Autodesk Inventor part; units mm, degrees
ref_plane "YZ Plane" through (0, 0, 0) normal (1, 0, 0) x (0, 1, 0)
ref_plane "XZ Plane" through (0, 0, 0) normal (0, 1, 0) x (-1, 0, 0)
ref_plane "XY Plane" through (0, 0, 0) normal (0, 0, 1) x (1, 0, 0)
sketch "Sketch1" plane through (0, 0, 0) normal (0, 0, 1) x (1, 0, 0)
  arc A0 (-6.0005, 54.2016) -> (-16.0004, 64.2461) centre (-16.0004, 54.2461) ccw construction
  line L0 (-16.0004, 64.2461) -> (-44.425, 64.2461) construction
  line L1 (-44.425, 64.2461) -> (-109.442, 0.9553) construction
  line L2 (-109.442, 0.9553) -> (-102.1149, -16.5964) construction
  arc A1 (-102.1149, -16.5964) -> (-98.2137, -18.2187) centre (-99.3465, -15.4407) ccw construction
  arc A2 (-98.2137, -18.2187) -> (-94.934, -16.1156) centre (-102.2552, -8.3072) ccw construction
  arc A3 (-90.1342, -27.6135) -> (-94.934, -16.1156) centre (-85.3155, -18.8511) ccw construction
  arc A4 (-90.1342, -27.6135) -> (-93.9357, -28.4666) centre (-89.7305, -38.3096) ccw construction
  arc A5 (-93.9357, -28.4666) -> (-95.5255, -32.381) centre (-92.7571, -31.2253) ccw construction
  line L3 (-95.5255, -32.381) -> (-88, -50.4082) construction
  line L4 (-88, -50.4082) -> (88, -50.4082) construction
  line L5 (88, -50.4082) -> (95.5255, -32.381) construction
  arc A6 (95.5255, -32.381) -> (93.9357, -28.4666) centre (92.7571, -31.2253) ccw construction
  arc A7 (93.9357, -28.4666) -> (90.1342, -27.6135) centre (89.7305, -38.3096) ccw construction
  arc A8 (94.934, -16.1156) -> (90.1342, -27.6135) centre (85.3155, -18.8511) ccw construction
  arc A9 (94.934, -16.1156) -> (98.2137, -18.2187) centre (102.2552, -8.3072) ccw construction
  arc A10 (98.2137, -18.2187) -> (102.1149, -16.5964) centre (99.3465, -15.4407) ccw construction
  line L6 (102.1149, -16.5964) -> (109.442, 0.9553) construction
  line L7 (109.442, 0.9553) -> (44.425, 64.2461) construction
  line L8 (44.425, 64.2461) -> (16.0004, 64.2461) construction
  arc A11 (16.0004, 64.2461) -> (6.0005, 54.2016) centre (16.0004, 54.2461) ccw construction
  arc A12 (6.0005, 54.2016) -> (6.0352, 52.5653) centre (54.7865, 54.419) ccw construction
  arc A13 (-6.0352, 52.5653) -> (6.0352, 52.5653) centre (0, 44.5918) ccw construction
  arc A14 (-6.0352, 52.5653) -> (-6.0005, 54.2016) centre (-54.7865, 54.419) ccw construction
  line L9 (109.442, 0.9553) -> (88, -50.4082)
  line L10 (88, -50.4082) -> (-88, -50.4082)
  line L11 (-88, -50.4082) -> (-109.442, 0.9553)
  line L12 (-109.442, 0.9553) -> (-44.425, 64.2461)
  line L13 (-44.425, 64.2461) -> (-24.425, 64.2461)
  line L14 (109.442, 0.9553) -> (95.1109, 14.9059)
  line L15 (-24.425, 60.2461) -> (-42.7995, 60.2461)
  line L16 (-42.7995, 60.2461) -> (-104.7029, -0.0138)
  line L17 (-104.7029, -0.0138) -> (-85.3353, -46.4082)
  line L18 (-85.3353, -46.4082) -> (85.3353, -46.4082)
  line L19 (85.3353, -46.4082) -> (104.7029, -0.0138)
  line L20 (104.7029, -0.0138) -> (92.3208, 12.0397)
  line L21 (92.3208, 12.0397) -> (95.1109, 14.9059)
  line L22 (-24.425, 60.2461) -> (-24.425, 64.2461)
  point P0 (0, 0)
  dimension "d1" = 20
  dimension "d2" = 20
  dimension "d3" = 4
extrude "Extrusion1" add sketch "Sketch1" along normal blind 1000
ref_plane "Work Plane1" through (0, 0, 0) normal (0, 0, 1) x (1, 0, 0)
sketch "Sketch2" plane through (0, 0, 0) normal (0, 0, 1) x (1, 0, 0)
  line L0 (109.442, 0.9553) -> (44.425, 64.2461) construction
  line L1 (-16.0004, 64.2461) -> (-44.425, 64.2461)
  line L2 (-44.425, 64.2461) -> (-109.442, 0.9553)
  line L3 (-109.442, 0.9553) -> (-88, -50.4082)
  line L4 (-88, -50.4082) -> (88, -50.4082)
  line L5 (88, -50.4082) -> (109.442, 0.9553)
  line L6 (109.442, 0.9553) -> (95.1109, 14.9059)
  line L7 (95.1109, 14.9059) -> (92.3208, 12.0397)
  line L8 (92.3208, 12.0397) -> (104.7029, -0.0138)
  line L9 (104.7029, -0.0138) -> (85.3353, -46.4082)
  line L10 (85.3353, -46.4082) -> (-85.3353, -46.4082)
  line L11 (-85.3353, -46.4082) -> (-104.7029, -0.0138)
  line L12 (-104.7029, -0.0138) -> (-42.7995, 60.2461)
  line L13 (-42.7995, 60.2461) -> (-24.425, 60.2461)
  line L14 (-24.425, 60.2461) -> (-24.425, 64.2461)
  line L15 (-24.425, 64.2461) -> (-44.425, 64.2461)
  line L16 (109.442, 0.9553) -> (44.425, 64.2461)
  line L17 (44.425, 64.2461) -> (-44.425, 64.2461)
  line L18 (-44.425, 68.2461) -> (46.0504, 68.2461)
  line L19 (46.0504, 68.2461) -> (112.2321, 3.8215)
  line L20 (-44.425, 64.2461) -> (-44.425, 68.2461)
  line L21 (112.2321, 3.8215) -> (109.442, 0.9553)
  point P0 (0, 0)
  dimension "d6" = 4
extrude "Extrusion2" add sketch "Sketch2" along normal blind 1000 contours L1 L20 L18 L19 L21 L6 L16 L17
fillet "Fillet1" radius 6 3 edges at (88, -50.4082, 500) (-88, -50.4082, 500) (-109.442, 0.9553, 500)
fillet "Fillet2" radius 6 1 edges at (109.442, 0.9553, 500)
chamfer "Chamfer1" distance 1 angle 45 1 edges at (-44.425, 68.2461, 500)
properties part number "aluco de metro" material "Steel, Carbon"
Here's how the part is built. I have some questions about the finished solid (model axes, mm). A direction names the side the tool comes from. Give positions to 0.01 mm unless a question says otherwise; leave off trailing zeros. Loops run counter-clockwise (first coordinate to the right, second up) from the corner with the lowest first, then second, coordinate; pieces in that order, holes last. Notation, with made-up numbers: M 71,-18 L 98,-18 A24 cw 98,-3 Z; hole C 50.25,37 d8. An arc over 180 degrees is marked long. Put each result on its own line as item: value. Start each with the question number.
(1) I need wall thicknesses on line 1 along Y through (x, z) = (14.5, 741.5); line 2 along Y through (x, z) = (-25, 54); line 3 along X through (y, z) = (-22, 883). Which ranges of each line are inside material? Lowest first, please. Write a range as [from, to].
(2) I want a section at B-B on y = -13. Please give me the cut outline in (x, z).
(3) For faces 4 (the flat face through (94.9, -23.5, 493)), 5 (the flat face through (1, -48, 1000)), which set-ups out of +Z, -Z, +X, -X, +Y, -Y let a thin tool reach every point of the face, with its end or its side?
(4) I want a section at C-C on x = 59. Please give me the cut outline in (y, z).
(5) Will these pins go through, and if not, where does the flat tip stop? pin 1 Ø2 at (y, z) = (61.5, 607.5) entering from +X; pin 2 Ø1.5 at (y, z) = (52, 169) entering from -X; pin 3 Ø8 at (x, z) = (-66.5, 705.5) entering from +Y.
(6) If we mould it in two halves opening along X, with no side actions, what happens to faces 1 (the flat face through (-98.577, -25.072, 493)), 2 (the flat face through (1, -48, 0)), 3 (the flat face through (70.123, 39.231, 493))? For each: +X half, -X half, draft (parallel to the pull), parting line (faces both ways), or undercut.
(7) I want a section at A-A on z = 60. Please give me the cut outline in (x, y) (1 decimal), then the cut area to 3 significant figures.
Answer block:
1. line 1: [-50.41, -46.41], [64.25, 68.25]
1. line 2: [-50.41, -46.41], [60.25, 68.25]
1. line 3: [-99.86, -95.52], [95.52, 99.86]
2. outline: M -103.62,0 L -99.28,0 L -99.28,1000 L -103.62,1000 Z; M 99.28,0 L 103.62,0 L 103.62,1000 L 99.28,1000 Z
3. face 4: +Z, -Z
3. face 5: +Z, +X, -X, +Y, -Y
4. outline: M -50.41,0 L -46.41,0 L -46.41,1000 L -50.41,1000 Z; M 50.06,0 L 55.64,0 L 55.64,1000 L 50.06,1000 Z
5. pin 1: x = 54.01
5. pin 2: x = -57.78
5. pin 3: y = 46.65
6. face 1: -X half
6. face 2: draft
6. face 3: undercut
7. outline: M -107.9,-2.8 L -89.5,-46.7 A6 ccw -84,-50.4 L 84,-50.4 A6 ccw 89.5,-46.7 L 109,-0.1 A6 cw 110.2,1.8 L 112.2,3.8 L 46.1,68.2 L -43.4,68.2 L -44.4,67.2 L -44.4,64.2 L -106.5,3.8 A6 ccw Z; hole M -104.7,0 L -85.3,-46.4 L 85.3,-46.4 L 104.7,0 L 92.3,12 L 95.1,14.9 L 44.4,64.2 L -24.4,64.2 L -24.4,60.2 L -42.8,60.2 Z
7. area: 2,340 mm^2
